```python
from build123d import *

# Parameters (mm, degrees)
SKETCH1_R                            = 69.85
BOSS_EXTRUDE1_DEPTH                  = 3.048
F_17_64_0_26563_DIAMETER_HOLE1_D     = 6.747002
F_17_64_0_26563_DIAMETER_HOLE1_DEPTH = 16.51
F_17_64_0_26563_DIAMETER_HOLE1_TIP   = 2.027003899
F_5_32_0_15625_DIAMETER_HOLE1_D      = 3.96875
F_5_32_0_15625_DIAMETER_HOLE1_DEPTH  = 16.51
F_5_32_0_15625_DIAMETER_HOLE1_TIP    = 1.192332791
F_5_8_0_625_DIAMETER_HOLE1_D         = 15.875
F_5_8_0_625_DIAMETER_HOLE1_DEPTH     = 16.51
F_5_8_0_625_DIAMETER_HOLE1_TIP       = 4.769331164
F_7_64_0_10938_DIAMETER_HOLE1_D      = 2.778252
F_7_64_0_10938_DIAMETER_HOLE1_DEPTH  = 16.51
F_7_64_0_10938_DIAMETER_HOLE1_TIP    = 0.834671108


with BuildPart() as part:
    # Sketch1 → Boss-Extrude1 (new body)
    with BuildSketch(Plane(origin=(0, 0, 0), x_dir=(1, 0, 0), z_dir=(0, 1, 0))):
        with Locations(Location((0, 0, 0), (0, 0, 90))):
            Circle(SKETCH1_R)
    extrude(amount=BOSS_EXTRUDE1_DEPTH)

    # 17/64 (0.26563) Diameter Hole1
    with Locations(Plane(origin=(-43.779439924, 0, 36.735311894), x_dir=(0, 0, -1), z_dir=(0, -1, 0))):
        with Locations((0, 0), (0, 87.558879848), (65.872994861, 85.392363774), (65.872994861, 2.166516074), (75.470311894, 43.779439924)):
            Hole(F_17_64_0_26563_DIAMETER_HOLE1_D / 2, depth=F_17_64_0_26563_DIAMETER_HOLE1_DEPTH)
            with Locations((0, 0, -(F_17_64_0_26563_DIAMETER_HOLE1_DEPTH + F_17_64_0_26563_DIAMETER_HOLE1_TIP / 2))):  # 118° drill point
                Cone(0, F_17_64_0_26563_DIAMETER_HOLE1_D / 2, F_17_64_0_26563_DIAMETER_HOLE1_TIP, mode=Mode.SUBTRACT)

    # 5/32 (0.15625) Diameter Hole1
    with Locations(Plane(origin=(-29.6545, 0, 52.7685), x_dir=(0, 0, -1), z_dir=(0, -1, 0))):
        with Locations((0, 0), (0, 49.53), (105.537, 49.53), (105.537, 0)):
            Hole(F_5_32_0_15625_DIAMETER_HOLE1_D / 2, depth=F_5_32_0_15625_DIAMETER_HOLE1_DEPTH)
            with Locations((0, 0, -(F_5_32_0_15625_DIAMETER_HOLE1_DEPTH + F_5_32_0_15625_DIAMETER_HOLE1_TIP / 2))):  # 118° drill point
                Cone(0, F_5_32_0_15625_DIAMETER_HOLE1_D / 2, F_5_32_0_15625_DIAMETER_HOLE1_TIP, mode=Mode.SUBTRACT)

    # 5/8 (0.625) Diameter Hole1
    with Locations(Plane(origin=(-42.818743744, 0, 7.525311894), x_dir=(0, 0, -1), z_dir=(0, -1, 0))):
        with Locations((0, 0), (-33.02, 37.929243744), (0, 85.637487488)):
            Hole(F_5_8_0_625_DIAMETER_HOLE1_D / 2, depth=F_5_8_0_625_DIAMETER_HOLE1_DEPTH)
            with Locations((0, 0, -(F_5_8_0_625_DIAMETER_HOLE1_DEPTH + F_5_8_0_625_DIAMETER_HOLE1_TIP / 2))):  # 118° drill point
                Cone(0, F_5_8_0_625_DIAMETER_HOLE1_D / 2, F_5_8_0_625_DIAMETER_HOLE1_TIP, mode=Mode.SUBTRACT)

    # 7/64 (0.10938) Diameter Hole1
    with Locations(Plane(origin=(-23.3045, 0, 17.182317033), x_dir=(0, 0, -1), z_dir=(0, -1, 0))):
        with Locations((0, 0), (38.7, 0)):
            Hole(F_7_64_0_10938_DIAMETER_HOLE1_D / 2, depth=F_7_64_0_10938_DIAMETER_HOLE1_DEPTH)
            with Locations((0, 0, -(F_7_64_0_10938_DIAMETER_HOLE1_DEPTH + F_7_64_0_10938_DIAMETER_HOLE1_TIP / 2))):  # 118° drill point
                Cone(0, F_7_64_0_10938_DIAMETER_HOLE1_D / 2, F_7_64_0_10938_DIAMETER_HOLE1_TIP, mode=Mode.SUBTRACT)


solid = part.part
```
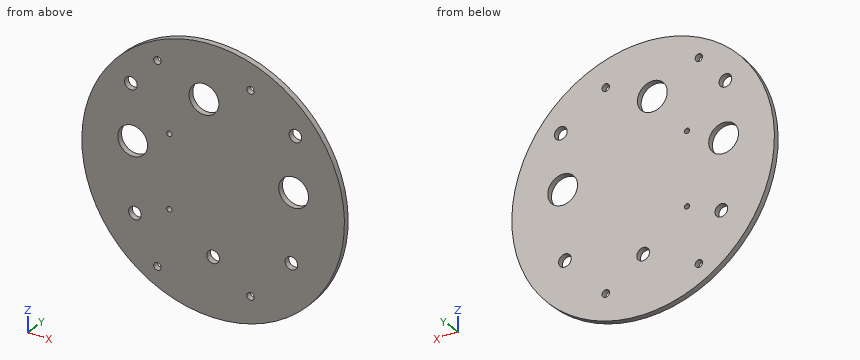
Geometry check sheet. Reference: the model listing, model coordinates, mm. Give positions to 0.01 mm unless a question says otherwise; leave off trailing zeros. Write each loop counter-clockwise with the first axis right and the second up, starting at its lowest first coordinate (ties: lowest second). Pieces come first, ordered by that corner, then holes.
1) Section check B-B, the plane y = 1.6. State how many separate pieces and enclosed holes the cut face has, and give its area (3 significant figures).
2) Material ranges on L1, parallel to X at y = 0.7, z = 2.5; L2, parallel to X at y = 2.05, z = 11.5; L3, parallel to X at y = 2.4, z = 35.5, recorded low to high.
3) Section check C-C, the plane z = 42. Record the boundary of the cut face in (x, y), and give its area (3 significant figures).
4) Section check D-D, the plane x = 53. Record the boundary of the cut face in (y, z), and give its area (3 significant figures).
5) Section check A-A, the plane x = 0. Record the boundary of the cut face in (y, z), and give its area (3 significant figures).
6) Gauge pin test, flat ends, axial feed: pin 1 (3.5 mm diameter, centred on x = -29.65, z = 52.77, fed in from +Y); pin 2 (1 mm diameter, centred on x = -35, y = 2, fed in from +Z). Record the tip position at first contact, or that the pin passes through.
Computed:
1. separate pieces: 1
1. enclosed holes: 14
1. area: 14,500 mm2
2. L1: x = -69.81 to -48.96, -36.67 to 36.67, 48.96 to 69.81
2. L2: x = -68.9 to -49.69, -35.95 to 35.95, 49.69 to 68.9
2. L3: x = -60.16 to -46.92, -40.64 to -11.02, 1.24 to 40.64, 46.92 to 60.16
3. outline: (-55.81, 0) - (-12.69, 0) - (-12.69, 3.05) - (-55.81, 3.05) - close; (2.91, 0) - (55.81, 0) - (55.81, 3.05) - (2.91, 3.05) - close
3. area: 293 mm2
4. outline: (0, -45.5) - (3.05, -45.5) - (3.05, 45.5) - (0, 45.5) - close
4. area: 277 mm2
5. outline: (0, -69.85) - (3.05, -69.85) - (3.05, -42.11) - (0, -42.11) - close; (0, -35.36) - (3.05, -35.36) - (3.05, 34.29) - (0, 34.29) - close; (0, 46.8) - (3.05, 46.8) - (3.05, 69.85) - (0, 69.85) - close
5. area: 367 mm2
6. pin 1: passes through
6. pin 2: stops at z = 60.74
